Input: part model. Units: mm. Frame: model coordinates. A direction names the side the tool comes from. Coordinates: 2 decimals unless noted, no trailing zeros. Write each loop counter-clockwise with the first axis right and the second up, starting at its lowest first coordinate (ties: lowest second). Pieces come first, ordered by that corner, then holes. Notation, with made-up numbers: (71, 8) - (92, 8) arc R24 cw to (92, 38) - close; hole circle Ø6 at (-25, 80.5). An arc over 180 degrees is marked (long way). Put each result on its own line as item: value. Start each with the question number.
1. Cut plane A-A, the plane z = 25. Return loops of the section in (x, y).
2. Access query for faces 5 (the flat face through (37.5, 0, 74)), 6 (the flat face through (27.5, -17, 125)), 7 (the flat face through (-27.5, -17, 25)). Directions: +Z, -Z, +X, -X, +Y, -Y. A direction counts if a zero-diameter tool reaches every point of the face in a straight line with its end or side. Return the directions, or none.
3. Pull-direction query (Y, two-part tool) for faces 1 (the cylindrical face through (32.57, -14.73, 124.09)), 2 (the cylindrical face through (-32.43, -14.73, 125.91)), 3 (the flat face through (-1, -25, 74)), 4 (the flat face through (-37.5, 0, 74)); classes: released by +Y, released by -Y, zero draft, split by the parting line, or undercut.
4. Line query: line 1 (Y direction, x = -35, z = 125). Output: solid intervals per line, ascending.
5. Pin query (flat end, axial travel): pin 1 (5 mm diameter, centred on y = -17, z = 126, fed in from -X); pin 2 (4 mm diameter, centred on y = -16.92, z = 125, fed in from -X). Return the tip coordinate at first contact, or that it passes through.
from build123d import *

# Parameters (mm, degrees)
SKETCH1_W           = 75
SKETCH1_H           = 50
BOSS_EXTRUDE1_DEPTH = 150
SKETCH2_R           = 2.369647205
CUT_EXTRUDE1_DEPTH  = 10
CUT_EXTRUDE2_START  = -10
SKETCH3_R           = 2.369647205
CUT_EXTRUDE2_DEPTH  = 10


with BuildPart() as part:
    # Sketch1 → Boss-Extrude1 (new body)
    with BuildSketch(Plane.XY):
        Rectangle(SKETCH1_W, SKETCH1_H)
    extrude(amount=BOSS_EXTRUDE1_DEPTH)

    # Sketch2 → Cut-Extrude1 (cut)
    with BuildSketch(Plane(origin=(37.5, 0, 0), x_dir=(0, 0, -1), z_dir=(1, 0, 0))):
        with Locations(Location((-125, -16.919154578, 0), (0, 0, 90))):
            Circle(SKETCH2_R)
        with Locations(Location((-25, -16.919154578, 0), (0, 0, 90))):
            Circle(SKETCH2_R)
    extrude(amount=-CUT_EXTRUDE1_DEPTH, mode=Mode.SUBTRACT)

    # Sketch3 → Cut-Extrude2 (cut)
    with BuildSketch(Plane.ZY.offset(37.5).offset(CUT_EXTRUDE2_START)):
        with Locations(Location((25, -16.919154578, 0), (0, 0, 90))):
            Circle(SKETCH3_R)
        with Locations(Location((125, -16.919154578, 0), (0, 0, 90))):
            Circle(SKETCH3_R)
    extrude(amount=CUT_EXTRUDE2_DEPTH, mode=Mode.SUBTRACT)


solid = part.part
Report:
1. outline: (-37.5, -25) - (37.5, -25) - (37.5, -19.29) - (27.5, -19.29) - (27.5, -14.55) - (37.5, -14.55) - (37.5, 25) - (-37.5, 25) - (-37.5, -14.55) - (-27.5, -14.55) - (-27.5, -19.29) - (-37.5, -19.29) - close
2. face 5: +Z, -Z, +X, +Y, -Y
2. face 6: +X
2. face 7: -X
3. face 1: undercut
3. face 2: undercut
3. face 3: released by -Y
3. face 4: zero draft
4. line 1: y = -25 to -19.29, -14.55 to 25
5. pin 1: stops at x = -37.5
5. pin 2: stops at x = -27.5
